```python
from build123d import *

# Parameters (mm, degrees)
F1_W     = 58.32
F1_H     = 61.06
F1_R     = 1.5
F2_DEPTH = 29.39
F8_W     = 129.0165177132
F8_H     = 143.0771122391
F3_W     = 31.47
F3_H     = 10.7


with BuildPart() as f2:
    # F1 (on offset) → F2 (new body)
    with BuildSketch(Plane.XY.offset(-12.64)):
        with Locations((0, 30.53)):
            Rectangle(F1_W, F1_H)
        with Locations((15.73, 16.46)):
            Circle(F1_R, mode=Mode.SUBTRACT)
        with Locations((-15.77, 46.69)):
            Circle(F1_R, mode=Mode.SUBTRACT)
        with Locations((-15.77, 46.69)):
            Circle(F1_R)
        with Locations((15.73, 16.46)):
            Circle(F1_R)
    extrude(amount=F2_DEPTH)

    # F8 (on offset) → F9 section 0
    with BuildSketch(Plane.XZ.offset(100)):
        Rectangle(F8_W, F8_H)
    # F3 (on face) → F9 section 1
    with BuildSketch(Plane.XZ):
        Rectangle(F3_W, F3_H)
    loft()


solid = f2.part
```
Can you work these out from the model? Positions are in its coordinate system, mm. A direction names the side the tool comes from. Coordinates: 2 decimals unless noted, no trailing zeros. Write each loop counter-clockwise with the first axis right and the second up, starting at its lowest first coordinate (ties: lowest second). Pieces come first, ordered by that corner, then holes. Notation, with made-up numbers: (-3, 5) - (53, 5) arc R35 ccw to (53, 38) - close; hole circle Ø11 at (69.25, 80). An arc over 180 degrees is marked (long way). Return JSON: item names as keys, results as strings.
Q1. Thinking about a two-plate mould opening in Y: for faces 1 (the flat face through (0, 31, 16.75)), 2 (the flat face through (0, 0, 8)), 3 (the flat face through (0, 61.06, 2)), which applies, +Y half, -Y half, draft (parallel to the pull), parting line (faces both ways), or undercut?
Computed values:
{"face 1": "draft", "face 2": "undercut", "face 3": "+Y half"}
Q2. I'm going to push flat-ended pins straight in: pin 1 Ø1 at (x, y) = (15.5, -81.5) entering from -Z; pin 2 Ø6 at (x, y) = (34, -73.5) entering from +Z; pin 3 Ø5 at (y, z) = (23.5, -7.5) entering from -X. Where does each tip first touch, or does it pass through?
Computed values:
{"pin 1": "stops at z = -59.62", "pin 2": "stops at z = 55.98", "pin 3": "stops at x = -29.16"}
Q3. Please list where these lines run through material, in increasing order: L1, parallel to Z at x = 29, y = 18; L2, parallel to Y at x = 16, z = 9.5; L3, parallel to X at y = -78.5, z = -42. Write a range as from..to.
Computed values:
{"L1": "z = -12.64..16.75", "L2": "y = -100..-6.27, 0..61.06", "L3": "x = -54.02..54.02"}
Q4. On a 3-axis mill with a long thin cutter (end or side, diameter ignored), from which of +Z, -Z, +X, -X, +Y, -Y can I reach the whole of each face in a straight line? I mean faces 4 (the flat face through (0, 31, -12.64)), 5 (the flat face through (29.16, 30, 2)), 6 (the flat face through (-2, -100, 0)), 7 (the flat face through (-29.16, 30, 2)). Say none if no direction works.
Computed values:
{"face 4": "-Z, +X, -X, +Y", "face 5": "+Z, -Z, +X, +Y", "face 6": "+Z, -Z, +X, -X, -Y", "face 7": "+Z, -Z, -X, +Y"}
Q5. If we section it at A-A (y = 8): Please give me the cut outline in (x, z), then the cut area to 3 significant figures.
Computed values:
{"outline": "(-29.16, -12.64) - (29.16, -12.64) - (29.16, 16.75) - (-29.16, 16.75) - close", "area": "1,710 mm2"}
